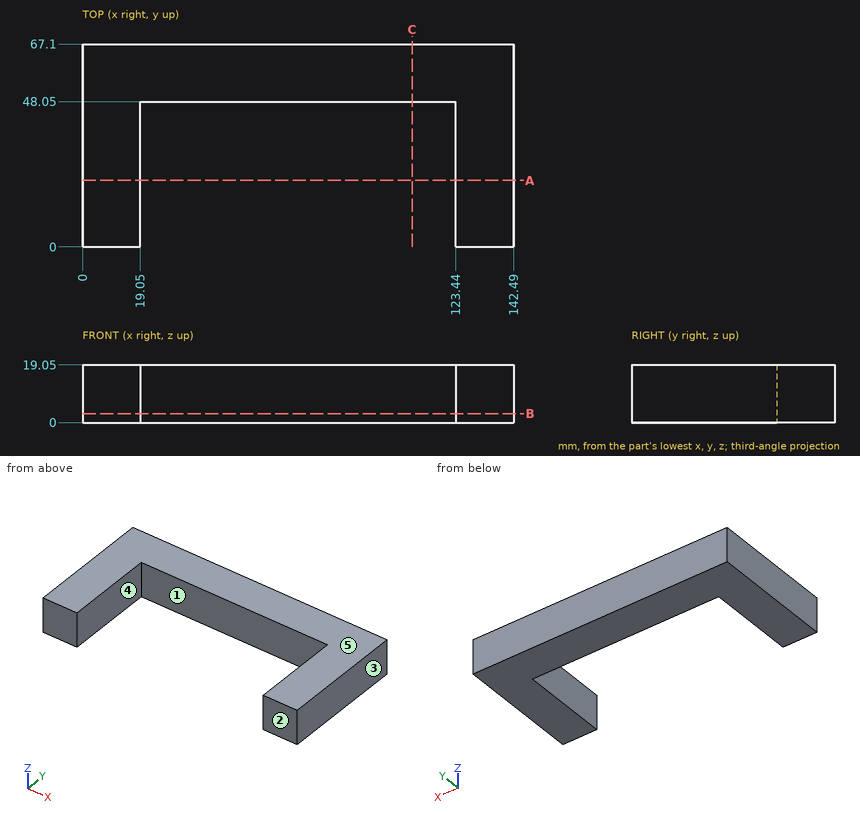
Here's the drawing with two shaded views (mm, measured from the low corner). I have some questions. A direction names the side the tool comes from. Give positions to 0.01 mm unless a question says otherwise; leave off trailing zeros. Loops run counter-clockwise (first coordinate to the right, second up) from the corner with the lowest first, then second, coordinate; pieces in that order, holes last. Notation, with made-up numbers: M 19,65.25 L 56,65.25 A26 ccw 56,79.25 Z; hole C 16,46 d4. An arc over 180 degrees is marked long. One line per item, written item: value.
1) I'm going to push a flat-ended pin straight in: pin 1 (5.5 mm diameter, centred on x = 90, z = 7.5, fed in from -Y). Where does the tip first touch, or does it pass through?
Geometry check:
pin 1: stops at y = 48.05
2) Please list where these lines run through material, in increasing order: line 1 (X direction, y = 12, z = 5.25); line 2 (Y direction, x = 96, z = 3).
Geometry check:
line 1: x = 0 to 19.05, 123.44 to 142.49
line 2: y = 48.05 to 67.1
3) Imagine slicing it at B-B on z = 3. Write out the boundary of the cut face in (x, y), and give its area (3 significant figures).
Geometry check:
outline: M 0,0 L 19.05,0 L 19.05,48.05 L 123.44,48.05 L 123.44,0 L 142.49,0 L 142.49,67.1 L 0,67.1 Z
area: 4,550 mm²
4) Imagine slicing it at C-C on x = 109. Write out the boundary of the cut face in (y, z), and give its area (3 significant figures).
Geometry check:
outline: M 48.05,0 L 67.1,0 L 67.1,19.05 L 48.05,19.05 Z
area: 363 mm²
5) On a 3-axis mill with a long thin cutter (end or side, diameter ignored), from which of +Z, -Z, +X, -X, +Y, -Y can I reach the whole of each face in a straight line? I mean the marked faces 4 and 5. Say none if no direction works.
Geometry check:
face 4: +Z, -Z, -Y
face 5: +Z, +X, -X, +Y, -Y
6) Imagine slicing it at A-A on y = 22. Write out the boundary of the cut face in (x, z), and give its area (3 significant figures).
Geometry check:
outline: M 0,0 L 19.05,0 L 19.05,19.05 L 0,19.05 Z; M 123.44,0 L 142.49,0 L 142.49,19.05 L 123.44,19.05 Z
area: 726 mm²
7) Thinking about a two-plate mould opening in X: for the marked faces 1, 2 and 3, which applies, +X half, -X half, draft (parallel to the pull), parting line (faces both ways), or undercut?
Geometry check:
face 1: undercut
face 2: draft
face 3: +X half
